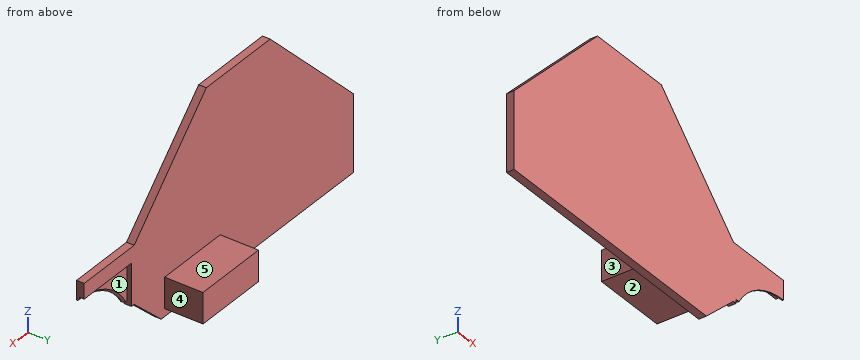
```python
from build123d import *

# Parameters (mm, degrees)
SALIENTE_EXTRUIR2_DEPTH = 2
CROQUIS3_W              = 17
CROQUIS3_H              = 11
CORTAR_EXTRUIR1_DEPTH   = 1.2
CORTAR_EXTRUIR2_DEPTH   = 1.8
CROQUIS5_W              = 20
CROQUIS5_H              = 8
SALIENTE_EXTRUIR3_DEPTH = 10
CHAFL_N1_SIZE           = 0.5


with BuildPart() as part:
    # Croquis1 → Saliente-Extruir2 (new body)
    with BuildSketch(Plane(origin=(0, 0, 0), x_dir=(1, 0, 0), z_dir=(0, 1, 0))):
        Polygon((0, 0), (0, 20), (69.25, 20), (79, 11), (97, 11), (97, -4), (79, -4), (53, -30), (30, -30), align=None)
    extrude(amount=SALIENTE_EXTRUIR2_DEPTH)

    # Croquis3 → Cortar-Extruir1 (cut)
    with BuildSketch(Plane(origin=(0, 2, 0), x_dir=(1, 0, 0), z_dir=(0, 1, 0))):
        with Locations((88.5, 5.5)):
            Rectangle(CROQUIS3_W, CROQUIS3_H)
    extrude(amount=-CORTAR_EXTRUIR1_DEPTH, mode=Mode.SUBTRACT)

    # Croquis4 → Cortar-Extruir2 (cut, through all)
    with BuildSketch(Plane(origin=(0, 0.8, 0), x_dir=(1, 0, 0), z_dir=(0, 1, 0))):
        with BuildLine():
            Line((80, 11), (80, 10))
            Line((80, 10), (81, 10))
            ThreePointArc((81, 10), (87.821220125, 3.404391333), (97, 1))
            Line((97, 1), (97, 11))
            Line((97, 11), (80, 11))
        make_face()
    extrude(amount=-CORTAR_EXTRUIR2_DEPTH, mode=Mode.SUBTRACT)

    # Croquis5 → Saliente-Extruir3 (add)
    with BuildSketch(Plane(origin=(0, 2, 0), x_dir=(1, 0, 0), z_dir=(0, 1, 0))):
        with Locations((58, 14)):
            Rectangle(CROQUIS5_W, CROQUIS5_H)
    extrude(amount=SALIENTE_EXTRUIR3_DEPTH)

    # Chaflán1
    chafl_n1_edges = [part.edges().sort_by_distance(p)[0] for p in [
        (87.821220125, 0.8, -3.404391333),
    ]]
    chamfer(chafl_n1_edges, length=CHAFL_N1_SIZE)


solid = part.part
```
Build history of the part. All positions in model axes, mm. Face numbers are marked on the shaded views. A direction names the side the tool comes from. Give positions to 0.01 mm unless a question says otherwise; leave off trailing zeros. Loops run counter-clockwise (first coordinate to the right, second up) from the corner with the lowest first, then second, coordinate; pieces in that order, holes last. Notation, with made-up numbers: (84, 44.25) - (95, 44.25) arc R17 ccw to (95, 61.25) - close; hole circle Ø2 at (-39, -29.75). An arc over 180 degrees is marked (long way). Use a Markdown table: item, result.
(1) Band-saw the part on B-B (x = 13). Give the cut face in (y, z), and give its area (3 significant figures).
Taken from the geometry:
| item | result |
|---|---|
| outline | (0, -20) - (2, -20) - (2, 13) - (0, 13) - close |
| area | 66.0 mm2 |
(2) Wall check: line 1 along Z through (x, y) = (53, 4.5); line 2 along X through (y, z) = (10.25, -12); line 3 along Y through (x, z) = (35.5, 2). Give the ranges that are in metal, low to high.
Taken from the geometry:
| item | result |
|---|---|
| line 1 | -18 to -10 |
| line 2 | 48 to 68 |
| line 3 | 0 to 2 |
(3) Band-saw the part on C-C (z = -12). Give the cut face in (x, y), and give its area (3 significant figures).
Taken from the geometry:
| item | result |
|---|---|
| outline | (0, 0) - (77.92, 0) - (77.92, 2) - (68, 2) - (68, 12) - (48, 12) - (48, 2) - (0, 2) - close |
| area | 356 mm2 |
(4) Which spindle directions (+Z, -Z, +X, -X, +Y, -Y) get a long thin tool onto all of the face, cutting with end or side? Do the marked faces 1, 2, 3, 4 and 5. Say none if no direction does.
Taken from the geometry:
| item | result |
|---|---|
| face 1 | -Z, +X, +Y |
| face 2 | -Z, +X, -X, +Y |
| face 3 | +Z, -Z, -X, +Y |
| face 4 | +Z, -Z, +X, +Y |
| face 5 | +Z, +X, -X, +Y |
(5) Drop flat-ended pins along their axis: pin 1 Ø5 at (x, z) = (37, -15) entering from +Y; pin 2 Ø6.5 at (y, z) = (8.5, -13) entering from +X; pin 3 Ø1.6 at (x, y) = (84, 1.5) entering from +Z; pin 4 Ø12 at (x, z) = (49, 12) entering from -Y. Give the stop position or say it passes through.
Taken from the geometry:
| item | result |
|---|---|
| pin 1 | y = 2 |
| pin 2 | x = 68 |
| pin 3 | z = 4 |
| pin 4 | y = 0 |
(6) Band-saw the part on A-A (z = 24). Give the cut face in (x, y), and give its area (3 significant figures).
Taken from the geometry:
| item | result |
|---|---|
| outline | (24, 0) - (59, 0) - (59, 2) - (24, 2) - close |
| area | 70.0 mm2 |
